```python
from build123d import *

# Parameters (mm, degrees)
IZIM1_W                     = 100
IZIM1_H                     = 35
Y_KSEKLIK_EKSTR_ZYON1_DEPTH = 35
RADYUS1_R                   = 17.5
RADYUS2_R                   = 17.5
RADYUS3_R                   = 17.5
IZIM2_R                     = 5
KES_EKSTR_ZYON1_DEPTH       = 64.492125496
PAH2_SIZE                   = 10
PAH3_SIZE                   = 10


# Some blends are built 0.0001 mm under size
with BuildPart() as part:
    # Çizim1 → Yükseklik-Ekstrüzyon1 (new body)
    with BuildSketch(Plane.XY):
        Rectangle(IZIM1_W, IZIM1_H)
    extrude(amount=Y_KSEKLIK_EKSTR_ZYON1_DEPTH)

    # Radyus1
    radyus1_edges = [part.edges().sort_by_distance(p)[0] for p in [
        (-50, 17.5, 17.5),
    ]]
    fillet(radyus1_edges, radius=RADYUS1_R)

    # Radyus2
    radyus2_edges = [part.edges().sort_by_distance(p)[0] for p in [
        (-50, -17.5, 17.5),
    ]]
    fillet(radyus2_edges, radius=RADYUS2_R - 0.0001)  # a hair under: the kernel refuses the full size

    # Radyus3
    radyus3_edges = [part.edges().sort_by_distance(p)[0] for p in [
        (50, -17.5, 17.5),
        (50, 17.5, 17.5),
    ]]
    fillet(radyus3_edges, radius=RADYUS3_R - 0.0001)  # a hair under: the kernel refuses the full size

    # Çizim2 → Kes-Ekstrüzyon1 (cut, through all)
    with BuildSketch(Plane.XY.offset(35)):
        with Locations((-50, 0)):
            Circle(IZIM2_R)
        with Locations((50, 0)):
            Circle(IZIM2_R)
    extrude(amount=-KES_EKSTR_ZYON1_DEPTH, mode=Mode.SUBTRACT)

    # Pah2
    # the kernel refuses this chamfer: 10 mm, written as the material it takes off along each edge
    with BuildSketch(Plane(origin=(-58.21682988, 17.5, 0), x_dir=(0, -0.9996219169112968, -0.027495876610586372), z_dir=(1, 0, 0))) as pah2_piece_1:
        Polygon((PAH2_SIZE * 0.999621916911, -PAH2_SIZE * 0.0274958766106), (-PAH2_SIZE * 0.0274958766106, -PAH2_SIZE * 0.999621916911), (0, 0), align=None)
    extrude(amount=116.433759759, mode=Mode.SUBTRACT)

    # Pah3
    # the kernel refuses this chamfer: 10 mm, written as the material it takes off along each edge
    with BuildSketch(Plane(origin=(58.21692988, -17.5, 0), x_dir=(0, 0.9996219169112968, -0.027495876610586372), z_dir=(-1, 0, 0)), Plane(origin=(58.21692988, -17.5, 35), x_dir=(0, -0.027495876610586317, -0.9996219169112968), z_dir=(-1, 0, 0))) as pah3_piece_1:
        Polygon((PAH3_SIZE * 0.999621916911, -PAH3_SIZE * 0.0274958766106), (-PAH3_SIZE * 0.0274958766106, -PAH3_SIZE * 0.999621916911), (0, 0), align=None)
    extrude(amount=116.433859759, mode=Mode.SUBTRACT)
    with BuildSketch(Plane(origin=(-58.21682988, 17.5, 35), x_dir=(0, -0.9996219169112968, 0.027495876610586317), z_dir=(1, 0, 0))) as pah3_piece_2:
        Polygon((PAH3_SIZE * 0.999621916911, PAH3_SIZE * 0.0274958766106), (-PAH3_SIZE * 0.0274958766106, PAH3_SIZE * 0.999621916911), (0, 0), align=None)
    extrude(amount=116.433759759, mode=Mode.SUBTRACT)


solid = part.part
```
Could you check a few things on this model? Use its own coordinates, in mm. Coordinates: 2 decimals unless noted, no trailing zeros. Order: outer loops, then holes, each group sorted by start corner. A loop starts at its lowest first (then second) coordinate and runs counter-clockwise, first axis right, second up. Notation, with made-up numbers: M -8.5,44 L 17.5,44 A17 cw 17.5,76 Z; hole C 41.25,55 d9. An arc over 180 degrees is marked long. Use a Markdown table: item, result. Add a question column.
Q1. I'm going to push flat-ended pins straight in: pin 1 (12 mm diameter, centred on y = -12.5, z = 28.5, fed in from +X); pin 2 (2 mm diameter, centred on x = 2, y = 10.5, fed in from +Z); pin 3 (12 mm diameter, centred on x = -33, y = 9, fed in from -Z); pin 4 (6 mm diameter, centred on y = 8, z = 20, fed in from +X). Where does each tip first touch, or does it pass through?
Q2. I want a section at C-C on y = 10. List the corners of the cut face in (x, z) for me, then the cut area to 3 significant figures.
Q3. If I drill on L1, parallel to Y at x = -10, z = 30.5; L2, parallel to Y at x = 42, z = 32.5; L3, parallel to X at y = 10.5, z = 13.5, over which ranges is the centre line in solid material (lowest first)?
Q4. I want a section at D-D on y = -9.5. List the corners of the cut face in (x, z) for me, then the cut area to 3 significant figures.
Q5. I want a section at A-A on z = 20. List the corners of the cut face in (x, y) for me.
Q6. I want a section at B-B on x = 4. List the corners of the cut face in (y, z) for me, then the cut area to 4 significant figures.
Q7. We'd pull the mould along Y, two halves only. Please class faces 1 (the flat face through (0, -17.5, 17)), 2 (the cylindrical face through (45, 0, 18)), 3 (the cylindrical face through (-45, 0, 18)), 4 (the flat face through (-0.7, 12.4, 30.1)): pulls with the +Y half, pulls with the -Y half, needs draft (parallel to the pull), parting line crosses it, or undercut.
Checked values:
| question | item | result |
|---|---|---|
| 1 | pin 1 | x = 48.75 |
| 1 | pin 2 | z = 33 |
| 1 | pin 3 | z = 0 |
| 1 | pin 4 | x = 49.27 |
| 2 | outline | M -46.86,2.5 L 46.86,2.5 L 46.86,32.5 L -46.86,32.5 Z |
| 2 | area | 2,810 mm² |
| 3 | L1 | -12 to 12 |
| 3 | L2 | -10 to 10 |
| 3 | L3 | -46.5 to 46.5 |
| 4 | outline | M -47.2,2 L 47.2,2 L 47.2,33 L -47.2,33 Z |
| 4 | area | 2,930 mm² |
| 5 | outline | M -49.29,-4.95 A17.5 ccw -32.5,-17.5 L 32.5,-17.5 A17.5 ccw 49.29,-4.95 A5 cw 49.29,4.95 A17.5 ccw 32.5,17.5 L -32.5,17.5 A17.5 ccw -49.29,4.95 A5 cw Z |
| 6 | outline | M -17.5,10 L -7.5,0 L 7.5,0 L 17.5,10 L 17.5,25 L 7.5,35 L -7.5,35 L -17.5,25 Z |
| 6 | area | 1,025 mm² |
| 7 | face 1 | pulls with the -Y half |
| 7 | face 2 | undercut |
| 7 | face 3 | undercut |
| 7 | face 4 | pulls with the +Y half |
